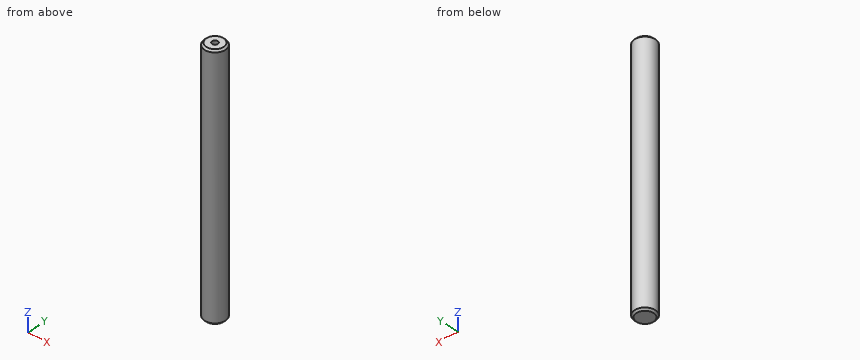
```python
from build123d import *

# Parameters (mm, degrees)
IZIM1_R                     = 4
Y_KSEKLIK_EKSTR_ZYON1_DEPTH = 96.6
IZIM3_R                     = 1.1
KES_EKSTR_ZYON2_DEPTH       = 25
PAH1_SIZE                   = 0.7
PAH2_SIZE                   = 0.7


with BuildPart() as part:
    # Çizim1 → Yükseklik-Ekstrüzyon1 (new body)
    with BuildSketch(Plane.XY):
        with Locations(Location((0, 0, 0), (0, 0, 180))):
            Circle(IZIM1_R)
    extrude(amount=Y_KSEKLIK_EKSTR_ZYON1_DEPTH)

    # Çizim3 → Kes-Ekstrüzyon2 (cut)
    with BuildSketch(Plane.XY.offset(96.6)):
        Circle(IZIM3_R)
    extrude(amount=-KES_EKSTR_ZYON2_DEPTH, mode=Mode.SUBTRACT)

    # Pah1
    pah1_edges = [part.edges().sort_by_distance(p)[0] for p in [
        (4, 0, 96.6),
    ]]
    chamfer(pah1_edges, length=PAH1_SIZE)

    # Pah2
    pah2_edges = [part.edges().sort_by_distance(p)[0] for p in [
        (4, 0, 0),
    ]]
    chamfer(pah2_edges, length=PAH2_SIZE)


solid = part.part
```
The model under review builds one solid part; all positions refer to its coordinate system, in mm. Round coordinates to 2 decimals unless told otherwise and drop trailing zeros. Loops run counter-clockwise (first coordinate to the right, second up) from the corner with the lowest first, then second, coordinate; pieces in that order, holes last.
Item 1: For line 1 (Y direction, x = 0, z = 84); line 2 (Y direction, x = -2.25, z = 59); line 3 (Z direction, x = -0.75, y = 0.5), list the stretches that pass through material, from the lowest coordinate up.
Determined:
line 1: y = -4 to -1.1, 1.1 to 4
line 2: y = -3.31 to 3.31
line 3: z = 0 to 71.6
Item 2: Clearance check with flat-ended pins moving along their axes: pin 1 Ø2 at (x, z) = (-2.5, 79) entering from +Y; pin 2 Ø1 at (y, z) = (-1.5, 78) entering from -X; pin 3 Ø2 at (x, y) = (0, 0) entering from +Z. State where each tip first meets the part, or that it passes through.
Determined:
pin 1: stops at y = 3.71
pin 2: stops at x = -3.87
pin 3: stops at z = 71.6
Item 3: Take a section at A-A (x = 0). Write out the cut boundary in (y, z).
Determined:
outline: (-4, 0.7) - (-3.3, 0) - (3.3, 0) - (4, 0.7) - (4, 95.9) - (3.3, 96.6) - (1.1, 96.6) - (1.1, 71.6) - (-1.1, 71.6) - (-1.1, 96.6) - (-3.3, 96.6) - (-4, 95.9) - close
Item 4: Take a section at D-D (z = 10.5). Write out the cut boundary in (x, y), then the cut area to 3 significant figures.
Determined:
outline: circle Ø8 at (0, 0)
area: 50.3 mm2
Item 5: Take a section at C-C (z = 73). Write out the cut boundary in (x, y).
Determined:
outline: circle Ø8 at (0, 0); hole circle Ø2.2 at (0, 0)
